Check sheet for the modelled part. Datum: model origin and axes. Units: mm. Round coordinates to 2 decimals unless told otherwise and drop trailing zeros. Loops run counter-clockwise (first coordinate to the right, second up) from the corner with the lowest first, then second, coordinate; pieces in that order, holes last. Notation, with made-up numbers: (-14, 29) -> (29, 29) arc R21 cw to (29, 54) -> close; hole circle Ø9 at (46, 83). An arc over 180 degrees is marked (long way). Use one line per item in the form item = value. Start each with the question number.
(1) Sectioned sample at A-A (y = 0). Record the cut outline in (x, z).
(2) Draft check along X on faces 1 (the cylindrical face through (432.386, 3.815, 25.044)), 2 (the cylindrical face through (-507.985, -1.396, 25.044)), 3 (the cylindrical face through (-456.614, 3.815, 25.044)), 4 (the cylindrical face through (507.985, 1.396, 25.044)). Enter one of: released by +X, released by -X, zero draft, split by the parting line, or undercut.
(3) Sectioned sample at B-B (z = 23). Record the cut outline in (x, y).
(4) Go/stop test with flat-tipped pins: pin 1 (4 mm diameter, centred on y = -16, z = 20.5, fed in from -X); pin 2 (4 mm diameter, centred on y = -28.5, z = 5.5, fed in from +X); pin 3 (2 mm diameter, centred on y = -41.5, z = 34, fed in from -X). Record where each tip stops, or that it passes through.
(5) Material ranges on probe 1 along X at (y, z) = (2, 32); probe 2 along Y at (x, z) = (444, 15); probe 3 along X at (y, z) = (-5.5, 37.5), recorded low to high. Write a range as [from, to].
(6) Sectioned sample at C-C (y = -49.5). Record the cut outline in (x, z), and give its area (3 significant figures).
from build123d import *

# Parameters (mm, degrees)
BOSS_EXTRUDE1_DEPTH = 50.8
SKETCH2_R           = 12.7
CUT_EXTRUDE1_DEPTH  = 515.467579153


with BuildPart() as part:
    # Sketch1 → Boss-Extrude1 (new body)
    with BuildSketch(Plane.XY):
        with BuildLine():
            Line((-444.5, 63.5), (444.5, 63.5))
            ThreePointArc((444.5, 63.5), (508, 0), (444.5, -63.5))
            Line((444.5, -63.5), (-444.5, -63.5))
            ThreePointArc((-444.5, -63.5), (-508, 0), (-444.5, 63.5))
        make_face()
    extrude(amount=BOSS_EXTRUDE1_DEPTH)

    # Sketch2 → Cut-Extrude1 (cut, through all)
    with BuildSketch(Plane(origin=(0, 0, 0), x_dir=(-1, 0, 0), z_dir=(0, 0, -1))):
        with Locations((444.5, 0)):
            Circle(SKETCH2_R)
        with Locations((-444.5, 0)):
            Circle(SKETCH2_R)
    extrude(amount=-CUT_EXTRUDE1_DEPTH, mode=Mode.SUBTRACT)


solid = part.part
Checks:
q1.outline = (-508, 0) -> (-457.2, 0) -> (-457.2, 50.8) -> (-508, 50.8) -> close; (-431.8, 0) -> (431.8, 0) -> (431.8, 50.8) -> (-431.8, 50.8) -> close; (457.2, 0) -> (508, 0) -> (508, 50.8) -> (457.2, 50.8) -> close
q2.face_1 = undercut
q2.face_2 = released by -X
q2.face_3 = undercut
q2.face_4 = released by +X
q3.outline = (-444.5, -63.5) -> (444.5, -63.5) arc R63.5 ccw to (444.5, 63.5) -> (-444.5, 63.5) arc R63.5 ccw to start; hole circle Ø25.4 at (-444.5, 0); hole circle Ø25.4 at (444.5, 0)
q4.pin_1 = -506.44
q4.pin_2 = 502.21
q4.pin_3 = -493.41
q5.probe_1 = [-507.97, -457.04], [-431.96, 431.96], [457.04, 507.97]
q5.probe_2 = [-63.5, -12.69], [12.69, 63.5]
q5.probe_3 = [-507.76, -455.95], [-433.05, 433.05], [455.95, 507.76]
q6.outline = (-484.27, 0) -> (484.27, 0) -> (484.27, 50.8) -> (-484.27, 50.8) -> close
q6.area = 49,200 mm2
